Model file for the job. Use its own axes, mm. Coordinates: 2 decimals unless noted, no trailing zeros. Loops run counter-clockwise (first coordinate to the right, second up) from the corner with the lowest first, then second, coordinate; pieces in that order, holes last.
from build123d import *

# Parameters (mm, degrees)
BOSS_EXTRUDE1_DEPTH = 25.4


with BuildPart() as part:
    # Sketch1 → Boss-Extrude1 (new body)
    with BuildSketch(Plane(origin=(0, 0, 0), x_dir=(1, 0, 0), z_dir=(0, 1, 0))):
        with BuildLine():
            Line((18.533658611, 35.641367486), (-39.99048208, 35.641367486))
            ThreePointArc((-39.99048208, 35.641367486), (-41.786533304, 34.89741871), (-42.53048208, 33.101367486))
            Line((-42.53048208, 33.101367486), (-42.53048208, -33.022533273))
            ThreePointArc((-42.53048208, -33.022533273), (-41.786533304, -34.818584498), (-39.99048208, -35.562533273))
            Line((-39.99048208, -35.562533273), (18.533658611, -35.562533273))
            ThreePointArc((18.533658611, -35.562533273), (20.329709835, -34.818584498), (21.073658611, -33.022533273))
            Line((21.073658611, -33.022533273), (21.073658611, -17.78))
            ThreePointArc((21.073658611, -17.78), (-27.572223111, 0), (21.073658611, 17.78))
            Line((21.073658611, 17.78), (21.073658611, 33.101367486))
            ThreePointArc((21.073658611, 33.101367486), (20.329709835, 34.89741871), (18.533658611, 35.641367486))
        make_face()
    extrude(amount=BOSS_EXTRUDE1_DEPTH)


solid = part.part
Q1. Slice it at C-C (y = 7.5). List the corners of the cut face in (x, z).
Answers:
outline: (-42.53, -33.1) arc R2.54 ccw to (-39.99, -35.64) - (18.53, -35.64) arc R2.54 ccw to (21.07, -33.1) - (21.07, -17.78) arc R27.57 cw (long way) to (21.07, 17.78) - (21.07, 33.02) arc R2.54 ccw to (18.53, 35.56) - (-39.99, 35.56) arc R2.54 ccw to (-42.53, 33.02) - close
Q2. Slice it at A-A (x = 0). List the corners of the cut face in (y, z).
Answers:
outline: (0, -35.64) - (25.4, -35.64) - (25.4, -27.57) - (0, -27.57) - close; (0, 27.57) - (25.4, 27.57) - (25.4, 35.56) - (0, 35.56) - close
Q3. Drill centre lines: line 1 (Z direction, x = -1, y = 9.25); line 2 (Z direction, x = 15.5, y = 12.25); line 3 (X direction, y = 15.5, z = -18). Where is each one in solid material? Low to high.
Answers:
line 1: z = -35.64 to -27.55, 27.55 to 35.56
line 2: z = -35.64 to -22.8, 22.8 to 35.56
line 3: x = -42.53 to -20.89, 20.89 to 21.07
Q4. Flat gauge pin, fed straight in: P1, Ø4, axis at y = 17, z = 5, coming from the +X side. Where does the tip first touch, or does it go through?
Answers:
P1: stops at x = -26.67
Q5. Slice it at B-B (z = -20). List the corners of the cut face in (x, y), and give its area (3 significant figures).
Answers:
outline: (-42.53, 0) - (-18.98, 0) - (-18.98, 25.4) - (-42.53, 25.4) - close; (18.98, 0) - (21.07, 0) - (21.07, 25.4) - (18.98, 25.4) - close
area: 651 mm2
Q6. Slice it at D-D (z = 0). List the corners of the cut face in (x, y), and give its area (3 significant figures).
Answers:
outline: (-42.53, 0) - (-27.57, 0) - (-27.57, 25.4) - (-42.53, 25.4) - close
area: 380 mm2
Q7. Mould opens along Z. For faces 1 (the flat face through (21.074, 13, 26)), 2 (the cylindrical face through (-27.556, 12.522, 0.942)), 3 (the flat face through (-11, 13, 35.563)) say: +Z half, -Z half, draft (parallel to the pull), parting line (faces both ways), or undercut.
Answers:
face 1: draft
face 2: undercut
face 3: +Z half
